Source: three-view drawing plus pictorial views. Frame: mm from the lowest corner of the part. A direction names the side the tool comes from. Give positions to 0.01 mm unless a question says otherwise; leave off trailing zeros. Loops run counter-clockwise (first coordinate to the right, second up) from the corner with the lowest first, then second, coordinate; pieces in that order, holes last. Notation, with made-up numbers: (-30.75, 53) - (-8.75, 53) arc R8 ccw to (-8.75, 67) - close; hole circle Ø7 at (54, 3). An arc over 180 degrees is marked (long way). Write each question's results on one line, items separated by ' | '. Start each with the question number.
(1) Pull-direction query (Z, two-part tool) for the marked faces 1, 2 and 3; classes: pulls with the +Z half, pulls with the -Z half, needs draft (parallel to the pull), parting line crosses it, or undercut.
(2) Cut plane B-B on z = 7.45. Return the cut outline in (x, y).
(3) Material intervals for line 1 along X through (y, z) = (3.75, 7.45); line 2 along Y through (x, z) = (2.1, 7.45); line 3 along Z through (x, y) = (8.5, 3.75), sorted ascending. Write a range as [from, to].
(4) Cut plane A-A on x = 7.45. Return the cut outline in (y, z), then the cut area to 3 significant figures.
(5) Cut plane D-D on z = 3.25. Return the cut outline in (x, y).
(6) Cut plane C-C on y = 5. Return the cut outline in (x, z), then the cut area to 3 significant figures.
(7) Contact query for flat-ended pins moving along their axis: pin 1 (1.6 mm diameter, centred on x = 7.45, y = 3, fed in from -Z); pin 2 (1.8 mm diameter, centred on y = 17, z = 7.45, fed in from -X); pin 3 (6 mm diameter, centred on x = 3.5, y = 2, fed in from +Z). Output: stop coordinate, or through.
(8) Reachability of the marked faces 4 and 5 from +Z, -Z, +X, -X, +Y, -Y: full face, straight path, thin tool, end or side. Return the list, or none.
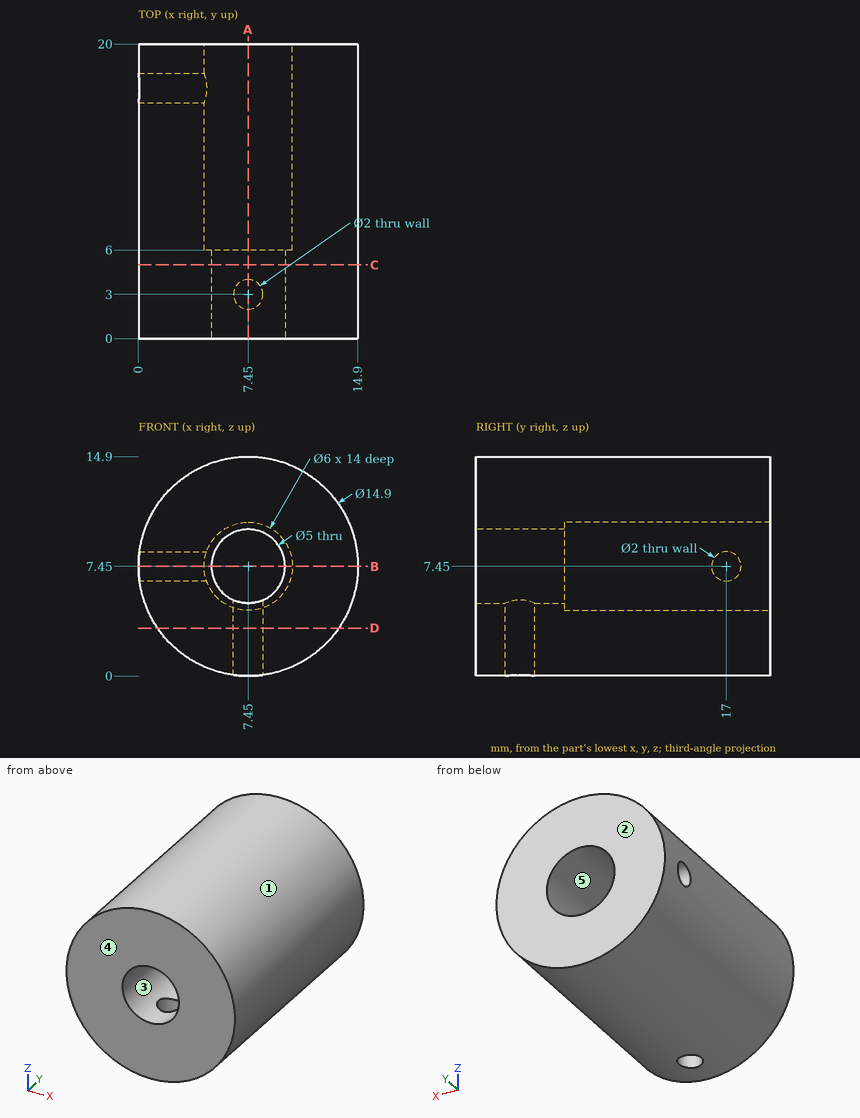
Ans:
1) face 1: parting line crosses it | face 2: needs draft | face 3: undercut
2) outline: (0, 0) - (4.95, 0) - (4.95, 6) - (4.45, 6) - (4.45, 16) - (0, 16) - close; (0, 18) - (4.45, 18) - (4.45, 20) - (0, 20) - close; (9.95, 0) - (14.9, 0) - (14.9, 20) - (10.45, 20) - (10.45, 6) - (9.95, 6) - close
3) line 1: [0, 4.95], [9.95, 14.9] | line 2: [0, 16], [18, 20] | line 3: [0.07, 5.18], [9.72, 14.83]
4) outline: (0, 0) - (2, 0) - (2, 4.95) - (0, 4.95) - close; (0, 9.95) - (6, 9.95) - (6, 10.45) - (20, 10.45) - (20, 14.9) - (0, 14.9) - close; (4, 0) - (20, 0) - (20, 4.45) - (6, 4.45) - (6, 4.95) - (4, 4.95) - close | area: 174 mm^2
5) outline: (1.3, 0) - (13.6, 0) - (13.6, 20) - (1.3, 20) - close; hole circle Ø2 at (7.45, 3)
6) outline: circle Ø14.9 at (7.45, 7.45); hole circle Ø5 at (7.45, 7.45) | area: 155 mm^2
7) pin 1: z = 9.82 | pin 2: x = 10.31 | pin 3: z = 14.84
8) face 4: +Z, -Z, +X, -X, -Y | face 5: +Y
